Geometry check sheet. Reference: drawing and pictorial views, mm from the part's lowest x, y, z. Round coordinates to 2 decimals unless told otherwise and drop trailing zeros. Loops run counter-clockwise (first coordinate to the right, second up) from the corner with the lowest first, then second, coordinate; pieces in that order, holes last. Notation, with made-up numbers: (66, 20.5) - (83, 20.5) arc R26 cw to (83, 49.5) - close; hole circle Ø9 at (24, -17.75). An arc over 180 degrees is marked (long way). Return JSON: item names as keys, results as strings.
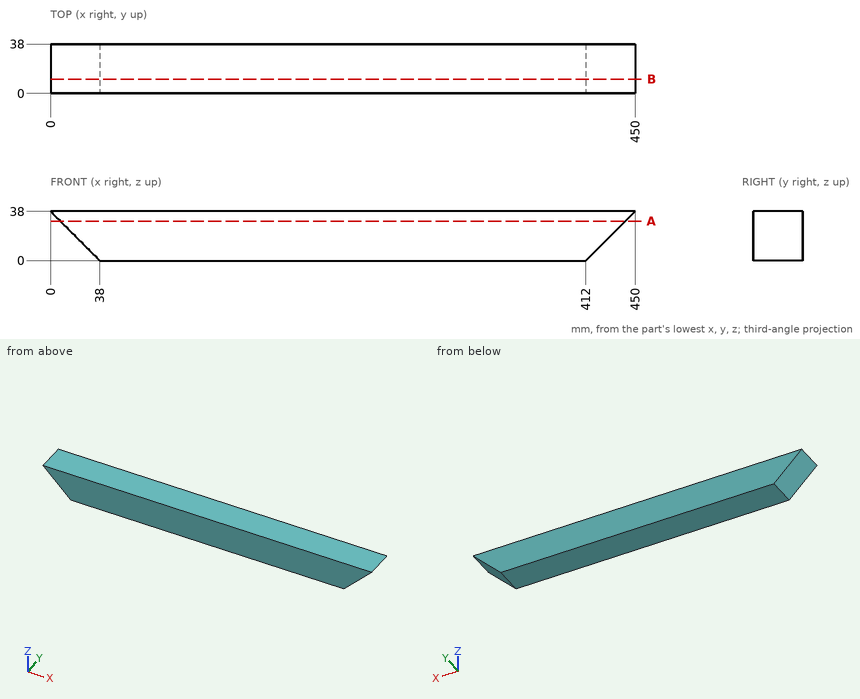
Q1. Sectioned sample at A-A (z = 30.5). Enter the section's corners in (x, y).
Answer key:
{"outline": "(7.5, 0) - (442.5, 0) - (442.5, 38) - (7.5, 38) - close"}
Q2. Scan lines: probe 1 along X at (y, z) = (18.5, 11.5); probe 2 along X at (y, z) = (24, 4). Record each from-to range of solid material in increasing order. Write a range as [from, to].
Answer key:
{"probe 1": "x = [26.5, 423.5]", "probe 2": "x = [34, 416]"}
Q3. Sectioned sample at B-B (y = 11). Enter the section's corners in (x, z).
Answer key:
{"outline": "(0, 38) - (38, 0) - (412, 0) - (450, 38) - close"}
Q4. Depth check by flat-ended pin: P1, Ø4, axis at y = 6.5, z = 8, coming from the -X side. Enter the tip coordinate at first touch or a pass-through.
Answer key:
{"P1": "stops at x = 28"}
